Source: three-view drawing plus pictorial views. Frame: mm from the lowest corner of the part. Give positions to 0.01 mm unless a question says otherwise; leave off trailing zeros. Loops run counter-clockwise (first coordinate to the right, second up) from the corner with the lowest first, then second, coordinate; pieces in that order, holes last. Notation, with made-up numbers: (20, -37.5) -> (51, -37.5) arc R10 ccw to (51, -24.5) -> close; hole circle Ø6 at (56.25, 15.5). An arc over 180 degrees is marked (long way). Answer in a Markdown table with one row per item. Add a question column.
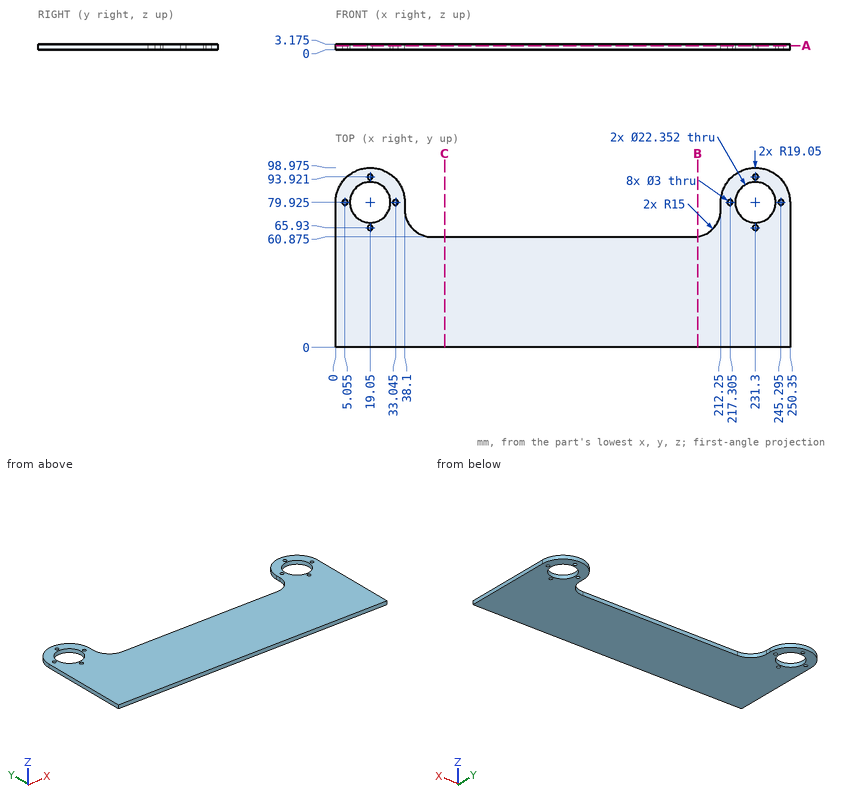
(1) Cut plane C-C on x = 60. Return the cut outline in (y, z) (1 decimal), then the cut area to 3 significant figures.
(2) Material intervals for line 1 along Y through (x, z) = (231, 0.6); line 2 along X through (y, z) = (94.5, 1.75) (1 decimal); line 3 along Y through (x, z) = (70, 1.35) (1 decimal), sorted ascending. Write a range as from..to.
(3) Cut plane A-A on z = 2.25. State how many separate pieces and enclosed holes the cut face has, then the cut area to 3 significant figures.
(4) Pin query (flat end, axial travel): pin 1 Ø1 at (x, z) = (102, 1) entering from +Y (1 decimal). Return the tip coordinate at first contact, or that it passes through.
(5) Cut plane B-B on x = 199.5. Return the cut outline in (y, z) (1 decimal), then the cut area to 3 significant figures.
Answer list:
| question | item | result |
|---|---|---|
| 1 | outline | (0, 0) -> (60.9, 0) -> (60.9, 3.2) -> (0, 3.2) -> close |
| 1 | area | 193 mm² |
| 2 | line 1 | y = 0..64.46, 67.4..68.75, 91.1..92.45, 95.39..98.97 |
| 2 | line 2 | x = 6.8..17.7, 20.4..31.3, 219..229.9, 232.7..243.6 |
| 2 | line 3 | y = 0..60.9 |
| 3 | separate pieces | 1 |
| 3 | enclosed holes | 10 |
| 3 | area | 17,100 mm² |
| 4 | pin 1 | stops at y = 60.9 |
| 5 | outline | (0, 0) -> (61, 0) -> (61, 3.2) -> (0, 3.2) -> close |
| 5 | area | 194 mm² |
